from build123d import *

# Parameters (mm, degrees)
F0_R     = 12.7
F1_DEPTH = 25.4
F2_W     = 50.247877
F2_H     = 25.4
F3_DEPTH = 25.4


with BuildPart() as f1:
    # F0 (on Top) → F1 (new body)
    with BuildSketch(Plane.XY):
        with BuildLine():
            Line((29.928832, 21.836502), (-33.571168, 21.836502))
            Line((-33.571168, 21.836502), (-33.571168, -28.963498))
            Line((-33.571168, -28.963498), (29.928832, -28.963498))
            ThreePointArc((29.928832, -28.963498), (55.328832, -3.563498), (29.928832, 21.836502))
        make_face()
        with Locations((-8.171168, -3.563498)):
            Circle(F0_R, mode=Mode.SUBTRACT)
        with Locations((29.928832, -3.563498)):
            Circle(F0_R, mode=Mode.SUBTRACT)
    extrude(amount=F1_DEPTH)

    # F2 (on face) → F3 (join)
    with BuildSketch(Plane(origin=(-33.571168, 0, 0), x_dir=(0, -1, 0), z_dir=(-1, 0, 0))):
        with BuildLine():
            Line((-21.284379, 25.4), (28.963498, 25.4))
            Line((28.963498, 25.4), (28.963498, 62.787746))
            Line((28.963498, 62.787746), (28.963498, 75.487746))
            ThreePointArc((28.963498, 75.487746), (25.281452, 84.430145), (16.370348, 88.187297))
            Line((16.370348, 88.187297), (16.370348, 62.787746))
            ThreePointArc((16.370348, 62.787746), (3.839559, 50.256958), (-8.691229, 62.787746))
            Line((-8.691229, 62.787746), (-8.691229, 88.187297))
            ThreePointArc((-8.691229, 88.187297), (-17.602333, 84.430145), (-21.284379, 75.487746))
            Line((-21.284379, 75.487746), (-21.284379, 62.787746))
            Line((-21.284379, 62.787746), (-21.284379, 25.4))
        make_face()
        with Locations((3.83956, 12.7)):
            Rectangle(F2_W, F2_H)
    extrude(amount=F3_DEPTH)


solid = f1.part
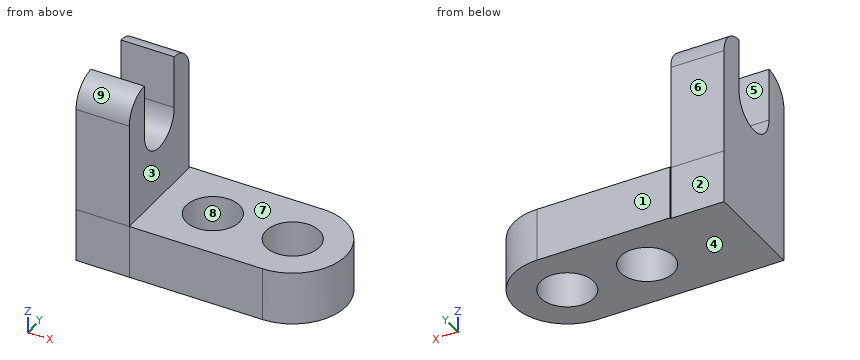
Can you work these out from the model? Positions are in its coordinate system, mm. Face numbers are marked on the shaded views. A direction names the side the tool comes from. Coordinates: 2 decimals unless noted, no trailing zeros. Order: outer loops, then holes, each group sorted by start corner. A loop starts at its lowest first (then second) coordinate and runs counter-clockwise, first axis right, second up. Notation, with made-up numbers: M -18.75,70 L 12.25,70 A24 ccw 12.25,88 Z; hole C -3,57 d1. An arc over 180 degrees is marked long. Answer as CSV lines item,"result".
(1) Suppose I cut it at D-D on x = -45. Please give me the cut outline in (y, z), plus the area to 3 significant figures.
Geometry check:
outline,"M -28.96,0 L 21.28,0 L 21.28,75.49 A12.7 ccw 8.69,88.19 L 8.69,62.79 A12.53 cw -16.37,62.79 L -16.37,88.19 A12.7 ccw -28.96,75.49 Z"
area,"3,480 mm^2"
(2) Suppose I cut it at A-A on z = 70. Please give me the cut outline in (x, y).
Geometry check:
outline,"M -58.97,-28.96 L -33.57,-28.96 L -33.57,-16.37 L -58.97,-16.37 Z; M -58.97,8.69 L -33.57,8.69 L -33.57,21.28 L -58.97,21.28 Z"
(3) Suppose I cut it at B-B on y = -12. Please give me the cut outline in (x, z), plus the area to 3 significant figures.
Geometry check:
outline,"M -58.97,0 L -17.66,0 L -17.66,25.4 L -33.57,25.4 L -33.57,53.28 L -58.97,53.28 Z; M 1.32,0 L 20.44,0 L 20.44,25.4 L 1.32,25.4 Z; M 39.42,0 L 53.89,0 L 53.89,25.4 L 39.42,25.4 Z"
area,"2,610 mm^2"
(4) Suppose I cut it at C-C on x = -8. Please give me the cut outline in (y, z), plus the area to 3 significant figures.
Geometry check:
outline,"M -28.96,0 L -16.26,0 L -16.26,25.4 L -28.96,25.4 Z; M 9.14,0 L 21.84,0 L 21.84,25.4 L 9.14,25.4 Z"
area,"645 mm^2"
(5) If we mould it in two halves opening along Y, with no side actions, what happens to the marked faces 6, 7, 8 and 9? For each: released by +Y, released by -Y, zero draft, split by the parting line, or undercut.
Geometry check:
face 6,"released by +Y"
face 7,"zero draft"
face 8,"undercut"
face 9,"released by -Y"
(6) I'm going to push flat-ended pins straight in: pin 1 (12 mm diameter, centred on x = 24.5, z = 32.5, fed in from -Y); pin 2 (20.5 mm diameter, centred on x = -42.5, z = 75, fed in from +Y); pin 3 (6 mm diameter, centred on y = -7, z = 17.5, fed in from +X); pin 4 (15 mm diameter, centred on y = -6, z = 56, fed in from +X). Where does each tip first touch, or does it pass through?
Geometry check:
pin 1,"through"
pin 2,"y = 21.28"
pin 3,"x = 55.33"
pin 4,"x = -33.57"
(7) Please list where these lines run through material, in increasing order: L1, parallel to X at y = 5.5, z = 10; L2, parallel to X at y = 15.5, z = 80; L3, parallel to Z at x = 22.5, y = 10.5.
Geometry check:
L1,"-58.97 to -17.07, 0.73 to 21.03, 38.83 to 53.66"
L2,"-58.97 to -33.57"
L3,"0 to 25.4"
(8) On a 3-axis mill with a long thin cutter (end or side, diameter ignored), from which of +Z, -Z, +X, -X, +Y, -Y can I reach the whole of each face in a straight line? I mean the marked faces 1, 2, 3, 4 and 5. Say none if no direction works.
Geometry check:
face 1,"+Z, -Z, +X, -X, +Y"
face 2,"+Z, -Z, -X, +Y"
face 3,"+Z, +X, +Y, -Y"
face 4,"-Z, +X, -X, +Y, -Y"
face 5,"+Z, +X, -X"
